Input: part model. Units: mm. Frame: model coordinates. A direction names the side the tool comes from. Round coordinates to 2 decimals unless told otherwise and drop trailing zeros. Loops run counter-clockwise (first coordinate to the right, second up) from the corner with the lowest first, then second, coordinate; pieces in that order, holes last. Notation, with made-up numbers: M -24,-20.5 L 32,-20.5 A19 cw 32,7.5 Z; hole C 61,30 d11. An arc over 180 degrees is marked long. Put each result on its own line as item: value. Start each with the question number.
1) Line query: probe 1 along X at (y, z) = (35, 6.25); probe 2 along Z at (x, y) = (70, 38); probe 3 along Y at (x, z) = (3.5, 1.5). Output: solid intervals per line, ascending.
2) Draft query along Y for faces 1 (the face through (53.845, 41, 6)), 2 (the face through (67.588, 30.226, 2.282)), 3 (the face through (-3, 0, -1)). Return one class per face: +Y half, -Y half, draft (parallel to the pull), parting line (faces both ways), or undercut.
3) Section A-A on x = 28. Output: boundary loops of the cut face in (y, z), plus the area to 3 significant figures.
4) Pin query (flat end, axial travel): pin 1 (6 mm diameter, centred on x = 8, z = 4.5, fed in from -Y); pin 2 (5 mm diameter, centred on x = 14, y = 35.5, fed in from -Z); pin 3 (1 mm diameter, centred on x = 9.5, y = 40, fed in from +Z); pin 4 (6 mm diameter, centred on x = 57, y = 23, fed in from -Z). Return the tip coordinate at first contact, or that it passes through.
5) Section C-C on x = 17. Output: boundary loops of the cut face in (y, z).
6) Reachability of faces 4 (the face through (-9.13, 22.18, 1.5)), 5 (the face through (37.81, 24.9, 4.06)), 6 (the face through (49, 42.5, 6)) from +Z, -Z, +X, -X, +Y, -Y: full face, straight path, thin tool, end or side. Return the list, or none.
7) Section B-B on z = 7. State how many separate pieces and enclosed holes the cut face has, plus the area to 3 significant figures.
from build123d import *

# Parameters (mm, degrees)
ESQUISSE1_R             = 2
BOSS_EXTRU_1_DEPTH      = 45
ESQUISSE2_W             = 75
ESQUISSE2_H             = 39
ENL_V_MAT_EXTRU_1_DEPTH = 8
ENL_V_MAT_EXTRU_2_DEPTH = 3.5
CONG_1_R                = 10
ESQUISSE4_W             = 20
ESQUISSE4_H             = 8
BOSS_EXTRU_2_DEPTH      = 15
CONG_3_R                = 3
ENL_V_MAT_EXTRU_3_DEPTH = 3.5
ESQUISSE6_R             = 2
ENL_V_MAT_EXTRU_4_DEPTH = 91.936473524


with BuildPart() as part:
    # Esquisse1 → Boss.-Extru.1 (new body)
    with BuildSketch(Plane(origin=(0, 0, 0), x_dir=(1, 0, 0), z_dir=(0, 1, 0))):
        Polygon((-13.665063509, 0.5), (-11.665063509, -2.964101615), (-6.531088913, 0), (3.665063509, 0), (3.665063509, -8), (78.665063509, -8), (78.665063509, 0), (8.665063509, 0), (8.665063509, 3), (-4.334936491, 3), align=None)
        with Locations(Location((49.844555434, -4, 0), (0, 0, 90))):
            Circle(ESQUISSE1_R, mode=Mode.SUBTRACT)
        with Locations(Location((9.844555434, -4, 0), (0, 0, 90))):
            Circle(ESQUISSE1_R, mode=Mode.SUBTRACT)
    extrude(amount=BOSS_EXTRU_1_DEPTH)

    # Esquisse2 → Enlèv. mat.-Extru.1 (cut)
    with BuildSketch(Plane.XY.offset(8)):
        with Locations((41.165063509, 19.5)):
            Rectangle(ESQUISSE2_W, ESQUISSE2_H)
    extrude(amount=-ENL_V_MAT_EXTRU_1_DEPTH, mode=Mode.SUBTRACT)

    # Esquisse3 → Enlèv. mat.-Extru.2 (cut)
    with BuildSketch(Plane.XZ.offset(-39)):
        Polygon((51.844555434, 0.535898385), (47.844555434, 0.535898385), (45.844555434, 4), (45.844555434, 8), (53.844555434, 8), (53.844555434, 4), align=None)
        Polygon((11.844555434, 0.535898385), (7.844555434, 0.535898385), (5.844555434, 4), (5.844555434, 8), (13.844555434, 8), (13.844555434, 4), align=None)
    extrude(amount=-ENL_V_MAT_EXTRU_2_DEPTH, mode=Mode.SUBTRACT)

    # Congé1
    # the kernel refuses this fillet: 10 mm, written as the material it adds along each edge
    with BuildSketch(Plane(origin=(3.665063509, 39, 0), x_dir=(-1, 0, 0), z_dir=(0, 1, 0))) as cong_1_piece_1:
        with BuildLine():
            CenterArc((9.797958971, 10), CONG_1_R, 191.536959033, 78.463040967)
            Line((0, 8), (-0.195959179, 7.96))
            ThreePointArc((-0.195959179, 7.96), (-0.2, 4), (-0.2, 0))
            Line((-0.2, 0), (0, -0.2))
            Line((0, -0.2), (9.797958971, -0.2))
            Line((9.797958971, -0.2), (9.797958971, 0))
        make_face()
    extrude(amount=6)

    # Esquisse4 → Boss.-Extru.2 (add)
    with BuildSketch(Plane.XZ.offset(-39)):
        with Locations((28.665063509, 4)):
            Rectangle(ESQUISSE4_W, ESQUISSE4_H)
        with Locations((66.665063509, 4)):
            Rectangle(ESQUISSE4_W, ESQUISSE4_H)
    extrude(amount=BOSS_EXTRU_2_DEPTH)

    # Congé3
    # the kernel refuses this fillet: 3 mm, written as the material it adds along each edge
    with BuildSketch(Plane(origin=(18.665063509, 39, 0), x_dir=(-1, 0, 0), z_dir=(0, 0, 1)), Plane(origin=(38.665063509, 39, 8), x_dir=(1, 0, 0), z_dir=(0, 0, -1))) as cong_3_piece_1:
        with BuildLine():
            CenterArc((CONG_3_R, CONG_3_R), CONG_3_R, 180, 90)
            Line((0, CONG_3_R), (0, 0))
            Line((0, 0), (CONG_3_R, 0))
        make_face()
    extrude(amount=8)
    with BuildSketch(Plane(origin=(76.665063509, 39, 8), x_dir=(1, 0, 0), z_dir=(0, 0, -1))) as cong_3_piece_2:
        with BuildLine():
            CenterArc((3, 2.828427125), CONG_3_R, 180, 70.528779366)
            Line((0, 2.828427125), (0, 0))
            Line((0, 0), (2, 0))
        make_face()
    extrude(amount=8)
    with BuildSketch(Plane(origin=(56.665063509, 39, 0), x_dir=(-1, 0, 0), z_dir=(0, 0, 1))) as cong_3_piece_3_section:
        with BuildLine():
            CenterArc((CONG_3_R, CONG_3_R), CONG_3_R, 180, 90)
            Line((0, CONG_3_R), (0, 0))
            Line((0, 0), (CONG_3_R, 0))
        make_face()
    cong_3_piece_3 = extrude(amount=8, mode=Mode.PRIVATE)
    cong_3_piece_3 = split(cong_3_piece_3, bisect_by=Plane(origin=(52.817631645, 39, 2.221315823), z_dir=(0.8660254037844395, 0, -0.4999999999999987)), keep=Keep.TOP, mode=Mode.PRIVATE)
    add(cong_3_piece_3)
    with BuildSketch(Plane(origin=(56.665063509, 39, -7.5), x_dir=(-1, 0, 0), z_dir=(0, 0, 1))) as cong_3_piece_4_section:
        with BuildLine():
            CenterArc((CONG_3_R, CONG_3_R), CONG_3_R, 180, 90)
            Line((0, CONG_3_R), (0, 0))
            Line((0, 0), (CONG_3_R, 0))
        make_face()
    cong_3_piece_4 = extrude(amount=15.5, mode=Mode.PRIVATE)
    cong_3_piece_4 = split(cong_3_piece_4, bisect_by=Plane(origin=(53.844555434, 39, -7.5), z_dir=(1, 0, 0)), keep=Keep.TOP, mode=Mode.PRIVATE)
    cong_3_piece_4 = split(cong_3_piece_4, bisect_by=Plane(origin=(49.570036381, 39, -3.403684177), z_dir=(-0.8660254037844395, 0, 0.4999999999999987)), keep=Keep.TOP, mode=Mode.PRIVATE)
    add(cong_3_piece_4)
    # the kernel refuses this fillet: 3 mm, written as the material it takes off along each edge
    with BuildSketch(Plane(origin=(76.665063509, 24, 15.5), x_dir=(-1, 0, 0), z_dir=(0, 0, -1)), Plane(origin=(18.665063509, 24, -7.5), x_dir=(1, 0, 0), z_dir=(0, 0, 1))) as cong_3_2_piece_1:
        with BuildLine():
            CenterArc((CONG_3_R, CONG_3_R), CONG_3_R, 180, 90)
            Line((0, CONG_3_R), (0, 0))
            Line((0, 0), (CONG_3_R, 0))
        make_face()
    extrude(amount=23, mode=Mode.SUBTRACT)
    with BuildSketch(Plane(origin=(56.665063509, 24, -7.5), x_dir=(0, 1, 0), z_dir=(0, 0, 1)), Plane(origin=(38.665063509, 24, 15.5), x_dir=(0, 1, 0), z_dir=(0, 0, -1))) as cong_3_2_piece_2:
        with BuildLine():
            CenterArc((CONG_3_R, -CONG_3_R), CONG_3_R, 90, 90)
            Line((0, -CONG_3_R), (0, 0))
            Line((0, 0), (CONG_3_R, 0))
        make_face()
    extrude(amount=23, mode=Mode.SUBTRACT)

    # Esquisse5 → Enlèv. mat.-Extru.3 (cut)
    with BuildSketch(Plane.XY.offset(8)):
        Polygon((32.665063509, 32), (30.665063509, 28.535898385), (26.665063509, 28.535898385), (24.665063509, 32), (26.665063509, 35.464101615), (30.665063509, 35.464101615), align=None)
        Polygon((70.665063509, 32), (68.665063509, 28.535898385), (64.665063509, 28.535898385), (62.665063509, 32), (64.665063509, 35.464101615), (68.665063509, 35.464101615), align=None)
    extrude(amount=-ENL_V_MAT_EXTRU_3_DEPTH, mode=Mode.SUBTRACT)

    # Esquisse6 → Enlèv. mat.-Extru.4 (cut, through all)
    with BuildSketch(Plane.XY.offset(4.5)):
        with Locations((28.665063509, 32)):
            Circle(ESQUISSE6_R)
        with Locations((66.665063509, 32)):
            Circle(ESQUISSE6_R)
    extrude(amount=-ENL_V_MAT_EXTRU_4_DEPTH, mode=Mode.SUBTRACT)


solid = part.part
Geometry results:
1. probe 1: x = 18.67 to 26.4, 30.93 to 38.67, 56.67 to 64.4, 68.93 to 76.67
1. probe 2: z = 0 to 8
1. probe 3: y = 39 to 45
2. face 1: draft
2. face 2: undercut
2. face 3: -Y half
3. outline: M 24,0 L 30.11,0 L 30.11,4.5 L 28.54,4.5 L 28.54,8 L 24,8 Z; M 33.89,0 L 45,0 L 45,8 L 35.46,8 L 35.46,4.5 L 33.89,4.5 Z
3. area: 127 mm²
4. pin 1: stops at y = 39
4. pin 2: passes through
4. pin 3: stops at z = 0.54
4. pin 4: stops at z = 0
5. outline: M 38.69,0 L 45,0 L 45,8 L 38.69,8 Z
6. face 4: +Z, +Y, -Y
6. face 5: +Z, -Z, -Y
6. face 6: +Z, -Y
7. separate pieces: 1
7. enclosed holes: 2
7. area: 912 mm²
